Geometry check sheet. Reference: drawing and pictorial views, mm from the part's lowest x, y, z. Give positions to 0.01 mm unless a question says otherwise; leave off trailing zeros. Write each loop counter-clockwise with the first axis right and the second up, starting at its lowest first coordinate (ties: lowest second). Pieces come first, ordered by that corner, then holes. Notation, with made-up numbers: (-37, 89) -> (-5, 89) arc R16 ccw to (-5, 111) -> close; hole circle Ø4 at (21, 81). An arc over 180 degrees is marked (long way). Use a Markdown table: item, result. Add a question column.
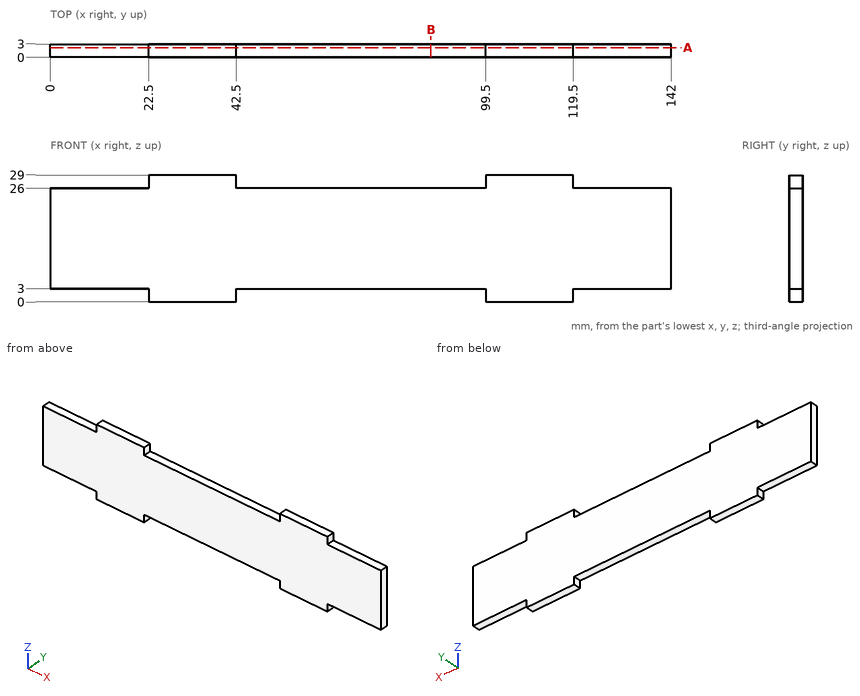
1) Sectioned sample at A-A, the plane y = 2.15. Enter the section's corners in (x, z), and give its area (3 significant figures).
2) Gauge pin test, flat ends, axial feed: P1, Ø0.9, axis at y = 1, z = 27, coming from the +X side; P2, Ø0.9, axis at x = 83.5, y = 2, coming from the +Z side; P3, Ø1.5, axis at x = 11, y = 1.5, coming from the -Z side; P4, Ø8, axis at x = 27.5, z = 20.5, coming from the -Y side. Record the tip position at first contact, or that the pin passes through.
3) Sectioned sample at B-B, the plane x = 87. Enter the section's corners in (y, z), and give its area (3 significant figures).
4) Material ranges on probe 1 along Z at (x, y) = (71.5, 1.7), recorded low to high. Write a range as [from, to].
Check values:
| question | item | result |
|---|---|---|
| 1 | outline | (0, 3) -> (22.5, 3) -> (22.5, 0) -> (42.5, 0) -> (42.5, 3) -> (99.5, 3) -> (99.5, 0) -> (119.5, 0) -> (119.5, 3) -> (142, 3) -> (142, 26) -> (119.5, 26) -> (119.5, 29) -> (99.5, 29) -> (99.5, 26) -> (42.5, 26) -> (42.5, 29) -> (22.5, 29) -> (22.5, 26) -> (0, 26) -> close |
| 1 | area | 3,510 mm² |
| 2 | P1 | x = 119.5 |
| 2 | P2 | z = 26 |
| 2 | P3 | z = 3 |
| 2 | P4 | y = 0 |
| 3 | outline | (0, 3) -> (3, 3) -> (3, 26) -> (0, 26) -> close |
| 3 | area | 69.0 mm² |
| 4 | probe 1 | [3, 26] |
